CAD build for the part. Positions are in the model's coordinates, mm. Face numbers are marked on the shaded views. A direction names the side the tool comes from. Round coordinates to 2 decimals unless told otherwise and drop trailing zeros. Loops run counter-clockwise (first coordinate to the right, second up) from the corner with the lowest first, then second, coordinate; pieces in that order, holes last.
from build123d import *

# Parameters (mm, degrees)
F0_W   = 3
F0_H   = 16
F2_W   = 58
F2_H   = 6.4001772553
F2_W_2 = 3
F2_H_2 = 12.5


with BuildPart() as f1:
    # F0 (on Front) → F1 (revolve)
    with BuildSketch(Plane.XZ):
        with BuildLine():
            Line((0, 0), (44, 0))
            Line((44, 0), (44, 31))
            Line((44, 31), (6, 31))
            ThreePointArc((6, 31), (1.7573593129, 29.2426406871), (0, 25))
            Line((0, 25), (0, 0))
        make_face()
        with BuildLine():
            Line((44, 0), (56, 0))
            Line((56, 0), (56, 31))
            ThreePointArc((56, 31), (50, 25), (44, 31))
            Line((44, 31), (44, 0))
        make_face()
        Polygon((56, 0), (68, 0), (68, 20), (68, 31), (56, 31), align=None)
        Polygon((68, 0), (85, 0), (85, 16), (85, 20), (68, 20), align=None)
        with Locations((86.5, 8)):
            Rectangle(F0_W, F0_H)
    revolve(axis=Axis((28, 0, 0), (-1, 0, 0)))

    # F2 (on Front) → F3 (revolve, cut)
    with BuildSketch(Plane.XZ):
        with Locations((59, 3.2000886276)):
            Rectangle(F2_W, F2_H)
        Polygon((22, 0), (30, 0), (30, 6.4001772553), (30, 16), (22, 16), align=None)
        Polygon((15, 0), (22, 0), (22, 16), (22, 20.5), (15, 20.5), (15, 12.5), align=None)
        with Locations((13.5, 6.25)):
            Rectangle(F2_W_2, F2_H_2)
        Polygon((1.5, 0), (12, 0), (12, 12.5), (12, 16), (1.5, 16), align=None)
        Polygon((0, 0), (1.5, 0), (1.5, 16), (1.5, 25), (0, 25), align=None)
    revolve(axis=Axis((74.5795071125, 0, 0), (1, 0, 0)), mode=Mode.SUBTRACT)


solid = f1.part
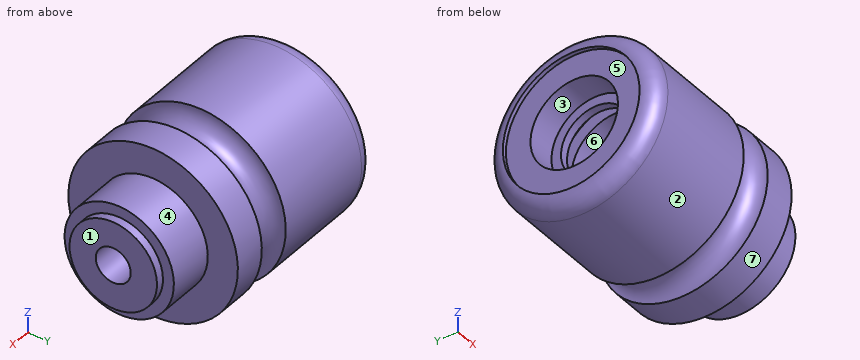
Item 1: Mould opens along Y. For the marked faces 1, 2 and 3 say: released by +Y, released by -Y, zero draft, split by the parting line, or undercut.
Verdict:
face 1: zero draft
face 2: split by the parting line
face 3: undercut
Item 2: Cut at B-B (x = 51). List the corners of the cut face in (y, z).
Verdict:
outline: circle Ø50.17 at (0, 0); hole circle Ø12.8 at (0, 0)
Item 3: 3-axis set-ups, long thin cutter, end or side, ignore diameter. For the marked faces 4, 5, 6 and 7: which of +Z, -Z, +X, -X, +Y, -Y reach the whole face in a straight line?
Verdict:
face 4: +X
face 5: -X
face 6: none
face 7: +X, -X
Item 4: Wall check: L1, parallel to Y at x = 10, z = 0; L2, parallel to X at y = -1, z = -13; L3, parallel to X at y = 5, z = -19. Give the ranges that are in metal, low to high.
Verdict:
L1: y = -31 to -16, 16 to 31
L2: x = 12 to 15, 30 to 88
L3: x = 1.5 to 15, 22 to 85
Item 5: Cut at A-A (x = 26). List the corners of the cut face in (y, z).
Verdict:
outline: circle Ø62 at (0, 0); hole circle Ø32 at (0, 0)
Item 6: Flat gauge pins, fed straight in: P1, Ø10, axis at x = 42.5, z = 18, coming from the +Y side; P2, Ø3, axis at x = 15.5, z = -24.5, coming from the +Y side; P3, Ø12, axis at x = 18, z = -2, coming from the -Y side. Where does each tip first touch, or does it go through?
Verdict:
P1: stops at y = 28.14
P2: stops at y = 20.78
P3: stops at y = -31
